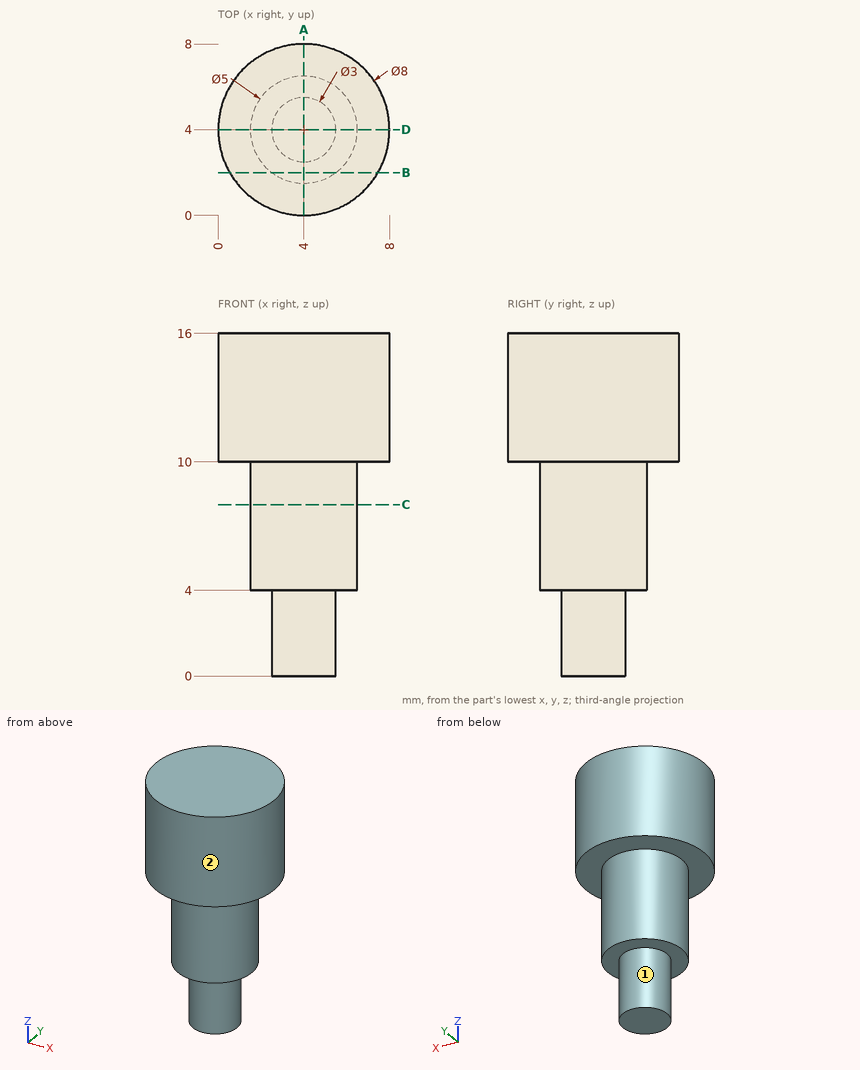
Answer from the drawing. Dimensions are ordinates in mm from the lowest x, y and z of the part. A direction names the side the tool comes from. Coordinates: 2 decimals unless noted, no trailing zeros. Loops run counter-clockwise (first coordinate to the right, second up) from the corner with the lowest first, then second, coordinate; pieces in that order, holes last.
Q1. The part is cut by section B-B on y = 2. Write down the section's boundary in (x, z), and give its area (3 significant figures).
Q2. This flat-tipped pin is pushed along its axis until it touches: pin 1 Ø2 at (y, z) = (6.5, 10) entering from -X. Where does it stop, or does it pass through?
Q3. The part is cut by section A-A on x = 4. Write down the section's boundary in (y, z).
Q4. The part is cut by section C-C on z = 8. Write down the section's boundary in (x, y), and give its area (3 significant figures).
Q5. Consider probe 1 along Z at (x, y) = (5.25, 7.25); probe 2 along Z at (x, y) = (3, 5.75); probe 3 along Y at (x, z) = (2, 6). Determine where each line is inside the solid, lowest interval first.
Q6. Which of the six approach directions +Z, -Z, +X, -X, +Y, -Y give full straight-line access (tool end or side, diameter ignored) to the marked faces 1 and 2?
Results below:
1. outline: (0.54, 10) - (2.5, 10) - (2.5, 4) - (5.5, 4) - (5.5, 10) - (7.46, 10) - (7.46, 16) - (0.54, 16) - close
1. area: 59.6 mm2
2. pin 1: stops at x = 0.29
3. outline: (0, 10) - (1.5, 10) - (1.5, 4) - (2.5, 4) - (2.5, 0) - (5.5, 0) - (5.5, 4) - (6.5, 4) - (6.5, 10) - (8, 10) - (8, 16) - (0, 16) - close
4. outline: circle Ø5 at (4, 4)
4. area: 19.6 mm2
5. probe 1: z = 10 to 16
5. probe 2: z = 4 to 16
5. probe 3: y = 2.5 to 5.5
6. face 1: -Z
6. face 2: +Z, -Z
